Check sheet for the modelled part. Datum: model origin and axes. Units: mm. A direction names the side the tool comes from. Round coordinates to 2 decimals unless told otherwise and drop trailing zeros. Write each loop counter-clockwise with the first axis right and the second up, starting at its lowest first coordinate (ties: lowest second). Pieces come first, ordered by that corner, then holes. Notation, with made-up numbers: M -29.5,-38.5 L -3.5,-38.5 A34 cw -3.5,-7.5 Z; hole C -28,-27 d3. An arc over 180 degrees is marked long. Answer in a Markdown table with one row per item.
```python
from build123d import *

# Parameters (mm, degrees)
F0_W      = 35
F0_H      = 10
F1_DEPTH  = 20
F3_DEPTH  = 25
F4_W      = 35
F4_H      = 5
F6_DEPTH  = 10.001
F7_DEPTH  = 10.001
F8_DEPTH  = 10.001
F9_R      = 3
F5_R      = 1.395
F10_DEPTH = 25
F5_R_2    = 4.25
F11_DEPTH = 112.584302492
F5_R_3    = 5.5
F12_DEPTH = 2


with BuildPart() as f1:
    # F0 (on Front) → F1 (new body)
    with BuildSketch(Plane.XZ):
        with BuildLine():
            Line((-0.9824314987, 41.1347855624), (-30.9824314987, -10.8267386647))
            Line((-30.9824314987, -10.8267386647), (64.0175685013, -10.8267386647))
            Line((64.0175685013, -10.8267386647), (64.0175685013, -0.8267386647))
            Line((64.0175685013, -0.8267386647), (57.0560442742, -0.8267386647))
            ThreePointArc((57.0560442742, -0.8267386647), (51.8796633722, -0.1452551905), (47.0560442742, 1.8527532596))
            Line((47.0560442742, 1.8527532596), (31.256660864, 10.9745315245))
            ThreePointArc((31.256660864, 10.9745315245), (30.5577721246, 11.8853410626), (30.7076227583, 13.0235696302))
            Line((30.7076227583, 13.0235696302), (31.2076227583, 13.889595034))
            Line((31.2076227583, 13.889595034), (13.8871146826, 23.889595034))
            Line((13.8871146826, 23.889595034), (13.3871146826, 23.0235696302))
            ThreePointArc((13.3871146826, 23.0235696302), (12.4763051446, 22.3246808908), (11.338076577, 22.4745315245))
            Line((11.338076577, 22.4745315245), (-3.3843552874, 30.9745315245))
            ThreePointArc((-3.3843552874, 30.9745315245), (-4.0832440268, 31.8853410626), (-3.933393393, 33.0235696302))
            Line((-3.933393393, 33.0235696302), (0.316606607, 40.3847855624))
            Line((0.316606607, 40.3847855624), (-0.9824314987, 41.1347855624))
        make_face()
        with BuildLine():
            ThreePointArc((-17.8532663741, -1.0863576079), (-20.1828955056, 1.9496741855), (-19.683393393, 5.743769411))
            Line((-19.683393393, 5.743769411), (-7.933393393, 26.0953663999))
            ThreePointArc((-7.933393393, 26.0953663999), (-4.8973615996, 28.4249955314), (-1.1032663741, 27.9254934189))
            Line((-1.1032663741, 27.9254934189), (47.2592382521, 0.0033883542))
            ThreePointArc((47.2592382521, 0.0033883542), (49.5888673835, -5.6208338902), (44.7592382521, -9.3267386647))
            Line((44.7592382521, -9.3267386647), (-3.5805077101, -9.3267386647))
            Line((-3.5805077101, -9.3267386647), (-17.8532663741, -1.0863576079))
        make_face(mode=Mode.SUBTRACT)
        with Locations((81.5175685013, -5.8267386647)):
            Rectangle(F0_W, F0_H)
    extrude(amount=F1_DEPTH)

    # F2 (on face) → F3 (cut)
    with BuildSketch(Plane(origin=(13.8162767634, 0, 23.9304933257), x_dir=(0.8660254038, 0, -0.5), z_dir=(0.5, 0, 0.8660254038))):
        with BuildLine():
            Line((13.5817965834, -6), (6.5817965834, -6))
            ThreePointArc((6.5817965834, -6), (2.5817965834, -10), (6.5817965834, -14))
            Line((6.5817965834, -14), (13.5817965834, -14))
            ThreePointArc((13.5817965834, -14), (17.5817965834, -10), (13.5817965834, -6))
        make_face()
    extrude(amount=-F3_DEPTH, mode=Mode.SUBTRACT)

    # F4 (on face) → F6 (cut, through all)
    with BuildSketch(Plane.XY.offset(-0.8267386647)):
        with Locations((81.5175685013, -2.5)):
            Rectangle(F4_W, F4_H)
    extrude(amount=-F6_DEPTH, mode=Mode.SUBTRACT)

    # F4 (on face) → F7 (cut, through all)
    with BuildSketch(Plane.XY.offset(-0.8267386647)):
        with Locations((81.5175685013, -17.5)):
            Rectangle(F4_W, F4_H)
    extrude(amount=-F7_DEPTH, mode=Mode.SUBTRACT)

    # F4 (on face) → F8 (cut, through all)
    with BuildSketch(Plane.XY.offset(-0.8267386647)):
        with BuildLine():
            Line((99.0175685013, -13), (99.0175685013, -7))
            Line((99.0175685013, -7), (82.0175685013, -7))
            ThreePointArc((82.0175685013, -7), (79.0175685013, -10), (82.0175685013, -13))
            Line((82.0175685013, -13), (99.0175685013, -13))
        make_face()
    extrude(amount=-F8_DEPTH, mode=Mode.SUBTRACT)

    # F9
    f9_edges = [f1.edges().sort_by_distance(p)[0] for p in [
        (64.017569, -5, -5.826739),
        (64.017569, -15, -5.826739),
    ]]
    fillet(f9_edges, radius=F9_R)

    # F5 (on face) → F10 (cut)
    with BuildSketch(Plane(origin=(-18.5487082622, 0, 10.7091017083), x_dir=(0, -1, 0), z_dir=(-0.8660254038, 0, 0.5))):
        with Locations((15, 7.1325535269)):
            Circle(F5_R)
        with Locations((15, 14.1325535269)):
            Circle(F5_R)
        with Locations((5, 14.1325535269)):
            Circle(F5_R)
        with Locations((5, 7.1325535269)):
            Circle(F5_R)
        with Locations((5, 0.1325535269)):
            Circle(F5_R)
        with Locations((15, 0.1325535269)):
            Circle(F5_R)
    extrude(amount=-F10_DEPTH, mode=Mode.SUBTRACT)

    # F5 (on face) → F11 (cut, through all)
    with BuildSketch(Plane(origin=(-18.5487082622, 0, 10.7091017083), x_dir=(0, -1, 0), z_dir=(-0.8660254038, 0, 0.5))):
        with Locations((10, -17.3674464731)):
            Circle(F5_R_2)
    extrude(amount=-F11_DEPTH, mode=Mode.SUBTRACT)

    # F5 (on face) → F12 (cut)
    with BuildSketch(Plane(origin=(-18.5487082622, 0, 10.7091017083), x_dir=(0, -1, 0), z_dir=(-0.8660254038, 0, 0.5))):
        with Locations((10, -17.3674464731)):
            Circle(F5_R_3)
        with Locations((10, -17.3674464731)):
            Circle(F5_R_2, mode=Mode.SUBTRACT)
    extrude(amount=-F12_DEPTH, mode=Mode.SUBTRACT)


solid = f1.part
```
1. Section check B-B, the plane z = 36.5. Record the cut outline in (x, y).
Found:
| item | result |
|---|---|
| outline | M -3.66,-20 L -1.93,-20 L -1.93,0 L -3.66,0 Z |
2. Section check C-C, the plane x = 54. Record the cut outline in (y, z), and give its area (3 significant figures).
Found:
| item | result |
|---|---|
| outline | M -20,-10.83 L 0,-10.83 L 0,-0.59 L -20,-0.59 Z |
| area | 205 mm2 |
3. Access from +Z, -Z, +X, -X, +Y, -Y to the whole of each face (thin tool, end or side, straight path). Record for faces 5 (the face through (-1.84, -9.86, 36.65)), 6 (the face through (91, -7, -6)), 7 (the face through (74, -10, -0.827)), 8 (the face through (-20.17, -9.86, 1.9)), 9 (the face through (15.067, -9.912, 20.931)).
Found:
| item | result |
|---|---|
| face 5 | +X, +Y, -Y |
| face 6 | +Z, -Z, +X |
| face 7 | +Z, +X, +Y, -Y |
| face 8 | +Y, -Y |
| face 9 | +X |
4. Draft check along Y on faces 1 (the face through (28.056, -10.088, 13.432)), 2 (the face through (-13.89, -9.86, 15.78)), 3 (the face through (13, -20, -10)), 4 (the face through (-17.32, -9.45, -5.19)). Enter one of: +Y half, -Y half, draft (parallel to the pull), parting line (faces both ways), or undercut.
Found:
| item | result |
|---|---|
| face 1 | undercut |
| face 2 | draft |
| face 3 | -Y half |
| face 4 | undercut |
5. Go/stop test with flat-tipped pins: pin 1 (1.5 mm diameter, centred on y = -11.5, z = 12.5, fed in from -X); pin 2 (3 mm diameter, centred on x = 91, z = -3.5, fed in from +Y); pin 3 (8 mm diameter, centred on x = 88.5, z = -8.5, fed in from -Y); pin 4 (10 mm diameter, centred on x = 32.5, z = 23.5, fed in from -Y). Record where each tip stops, or that it passes through.
Found:
| item | result |
|---|---|
| pin 1 | stops at x = -17.95 |
| pin 2 | stops at y = -5 |
| pin 3 | stops at y = -15 |
| pin 4 | passes through |
6. Scan lines: L1, parallel to Z at x = 0, y = -2.5; L2, parallel to X at y = -13, z = 3; L3, parallel to X at y = -8, z = 28. Record each from-to range of solid material in increasing order.
Found:
| item | result |
|---|---|
| L1 | z = -10.83 to -9.33, 27.29 to 29.02, 39.84 to 40.57 |
| L2 | x = -23 to -20.35, 42.07 to 45.07 |
| L3 | x = -8.57 to -5.97, -1.24 to 1.77 |
